Source: CAD feature listing. Evaluate the final solid. Frame: model axes, mm. Round coordinates to 2 decimals unless told otherwise and drop trailing zeros. Write each loop counter-clockwise with the first axis right and the second up, starting at its lowest first coordinate (ties: lowest second). Pieces come first, ordered by that corner, then holes. Notation, with made-up numbers: (-20.75, -3) -> (4.25, -3) arc R33 cw to (4.25, 32) -> close; hole circle Ø9 at (84, 3). An arc over 180 degrees is marked (long way). Put each result on its own line as item: value.
Autodesk Inventor part; units mm, degrees
ref_plane "YZ Plane" through (0, 0, 0) normal (1, 0, 0) x (0, 1, 0)
ref_plane "XZ Plane" through (0, 0, 0) normal (0, 1, 0) x (-1, 0, 0)
ref_plane "XY Plane" through (0, 0, 0) normal (0, 0, 1) x (1, 0, 0)
ref_plane "Work Plane1" through (0, 0, 0) normal (0, 0, 1) x (1, 0, 0)
sketch "Sketch1" plane through (0, 0, 0) normal (0, 0, 1) x (1, 0, 0)
  circle A0 centre (0, 0) radius 117.475
  point P0 (0, 0)
extrude "Extrusion1" add sketch "Sketch1" along normal blind -12.7
sketch "Sketch3" plane through (0, 0, -12.7) normal (0, 0, -1) x (-1, 0, 0)
  circle A0 centre (0, 0) radius 117.475
  circle A1 centre (0, 0) radius 6.35
  circle A2 centre (0, 0) radius 95.25
  circle A3 centre (0, 76.2) radius 19.05
  line L0 (34.6081, 88.7403) -> (14.8223, 64.2332)
  point P0 (0, 95.25)
  dimension "d15" = 12.7
  dimension "d16" = 38.1
extrude "Extrusion5" cut sketch "Sketch3" against normal through all contours A1 | L0 A3 A2 | A3 picked at (25.5173, 87.1725)
pattern_circular "Circular Pattern2" count 8 over 360 about axis through (0, 0, -12.7) along (0, 0, 1) of "Extrusion5"
properties part number "hubSpider" material "Wood (Maple)"
Q1. Material intervals for line 1 (Y direction, x = 0, z = -7.25) (3 decimals); line 2 (Y direction, x = -44.5, z = -4.5); line 3 (Y direction, x = 67, z = -7.75), sorted ascending. Write a range as [from, to].
Ans:
line 1: y = [-117.475, -95.25], [-57.15, -6.35], [6.35, 57.15], [95.25, 117.475]
line 2: y = [-108.72, -84.22], [-37.3, 37.3], [70.46, 108.72]
line 3: y = [-96.5, -67.69], [-36.12, -16.68], [17.06, 40.07], [67.7, 96.5]
Q2. Cut plane A-A on z = -7. Give the number of separate pieces and of enclosed holes in the cut face, and give its area (3 significant figures).
Ans:
separate pieces: 1
enclosed holes: 9
area: 32,000 mm^2
Q3. Cut plane B-B on y = -48.5. Output: boundary loops of the cut face in (x, z).
Ans:
outline: (-107, -12.7) -> (-72.16, -12.7) -> (-72.16, 0) -> (-107, 0) -> close; (-35.61, -12.7) -> (35.61, -12.7) -> (35.61, 0) -> (-35.61, 0) -> close; (81.98, -12.7) -> (107, -12.7) -> (107, 0) -> (81.98, 0) -> close
Q4. Pin query (flat end, axial travel): pin 1 (2 mm diameter, centred on y = 42.5, z = -4.5, fed in from -X); pin 2 (1.5 mm diameter, centred on y = -68.5, z = -4.5, fed in from -X); pin 3 (6 mm diameter, centred on y = 85, z = -3, fed in from -X). Return the tip coordinate at first contact, or that it passes through.
Ans:
pin 1: stops at x = -109.9
pin 2: stops at x = -95.97
pin 3: stops at x = -84.12
Q5. Cut plane D-D on x = 76.2. Output: boundary loops of the cut face in (y, z), and give its area (3 significant figures).
Ans:
outline: (-89.41, -12.7) -> (-57.15, -12.7) -> (-57.15, 0) -> (-89.41, 0) -> close; (-37.1, -12.7) -> (-19.05, -12.7) -> (-19.05, 0) -> (-37.1, 0) -> close; (24.48, -12.7) -> (89.41, -12.7) -> (89.41, 0) -> (24.48, 0) -> close
area: 1,460 mm^2
Q6. Cut plane C-C on x = -3. Output: boundary loops of the cut face in (y, z), and give its area (3 significant figures).
Ans:
outline: (-117.44, -12.7) -> (-95.01, -12.7) -> (-95.01, 0) -> (-117.44, 0) -> close; (-57.39, -12.7) -> (-5.6, -12.7) -> (-5.6, 0) -> (-57.39, 0) -> close; (5.6, -12.7) -> (57.39, -12.7) -> (57.39, 0) -> (5.6, 0) -> close; (95.2, -12.7) -> (117.44, -12.7) -> (117.44, 0) -> (95.2, 0) -> close
area: 1,880 mm^2
Q7. Draft query along X for faces 1 (the flat face through (24, 2, 0)), 2 (the cylindrical face through (93.562, 17.851, -6.439)), 3 (the cylindrical face through (-93.224, -71.482, -6.261)). Return one class per face: +X half, -X half, draft (parallel to the pull), parting line (faces both ways), or undercut.
Ans:
face 1: draft
face 2: undercut
face 3: parting line
